Autodesk Inventor part; units mm, degrees
ref_plane "YZ Plane" through (0, 0, 0) normal (1, 0, 0) x (0, 1, 0)
ref_plane "XZ Plane" through (0, 0, 0) normal (0, 1, 0) x (-1, 0, 0)
ref_plane "XY Plane" through (0, 0, 0) normal (0, 0, 1) x (1, 0, 0)
sketch "Sketch1" plane through (0, 0, 0) normal (0, 0, 1) x (1, 0, 0)
  circle A0 centre (-3.6979, 7.9302) radius 2.5 construction
  circle A1 centre (3.6979, -7.9302) radius 2.5 construction
  line L0 (-8.2294, 5.8171) -> (-0.8336, -10.0433) construction
  arc A2 (-0.8336, -10.0433) -> (8.2294, -5.8171) centre (3.6979, -7.9302) ccw construction
  line L1 (8.2294, -5.8171) -> (0.8336, 10.0433) construction
  arc A3 (0.8336, 10.0433) -> (-8.2294, 5.8171) centre (-3.6979, 7.9302) ccw construction
  circle A4 centre (78.5293, 90.1574) radius 2.5 construction
  circle A5 centre (94.3897, 82.7616) radius 2.5 construction
  line L2 (76.4162, 85.6259) -> (92.2766, 78.2301) construction
  arc A6 (92.2766, 78.2301) -> (96.5028, 87.2931) centre (94.3897, 82.7616) ccw construction
  line L3 (96.5028, 87.2931) -> (80.6424, 94.689) construction
  arc A7 (80.6424, 94.689) -> (76.4162, 85.6259) centre (78.5293, 90.1574) ccw construction
  circle A8 centre (-75.543, 162.0025) radius 75 construction
  line L4 (112.457, 50.5739) -> (112.457, -27.9975) construction
  line L5 (107.457, -32.9975) -> (39.927, -32.9975) construction
  line L6 (-75.543, 162.0025) -> (58.8073, 27.6522) construction
  line L7 (54.2111, 23.056) -> (63.4035, 32.2484)
  line L8 (70.4745, 32.2484) -> (91.6877, 11.0352)
  line L9 (54.2111, 15.985) -> (75.4243, -5.2282)
  line L10 (75.4243, -12.2993) -> (70.027, -17.6966)
  line L11 (98.7588, 11.0352) -> (104.1561, 16.4325)
  line L12 (-0.8336, -10.0433) -> (-8.2294, 5.8171)
  line L13 (80.6424, 94.689) -> (96.5028, 87.2931)
  arc A9 (-5.811, 12.4617) -> (73.9978, 92.2705) centre (-75.543, 162.0025) ccw
  line L14 (-3.6979, 7.9302) -> (3.6979, -7.9302) construction
  line L15 (78.5293, 90.1574) -> (94.3897, 82.7616) construction
  line L16 (65.9977, -19.1366) -> (3.2042, -12.9058)
  line L17 (105.5961, 20.4618) -> (99.3653, 83.2553)
  arc A10 (75.4243, -12.2993) -> (75.4243, -5.2282) centre (71.8887, -8.7638) ccw
  arc A11 (54.2111, 23.056) -> (54.2111, 15.985) centre (57.7466, 19.5205) ccw
  arc A12 (70.4745, 32.2484) -> (63.4035, 32.2484) centre (66.939, 28.7129) ccw
  arc A13 (91.6877, 11.0352) -> (98.7588, 11.0352) centre (95.2233, 14.5708) ccw
  arc A14 (104.1561, 16.4325) -> (105.5961, 20.4618) centre (100.6206, 19.9681) ccw
  arc A15 (99.3653, 83.2553) -> (96.5028, 87.2931) centre (94.3897, 82.7616) ccw
  arc A16 (80.6424, 94.689) -> (73.9978, 92.2705) centre (78.5293, 90.1574) ccw
  arc A17 (-5.811, 12.4617) -> (-8.2294, 5.8171) centre (-3.6979, 7.9302) ccw
  arc A18 (-0.8336, -10.0433) -> (3.2042, -12.9058) centre (3.6979, -7.9302) ccw
  arc A19 (65.9977, -19.1366) -> (70.027, -17.6966) centre (66.4914, -14.1611) ccw
  point P0 (0, 0)
  point P1 (79.4008, -9.1758)
  point P2 (50.6755, 19.5205)
  point P3 (66.939, 35.784)
  point P4 (95.2233, 7.4997)
  point P5 (78.9598, -8.7638)
  point P6 (68.3532, -19.3704)
  point P7 (105.8299, 18.1063)
  point P8 (0.37, -12.6245)
  point P9 (76.0422, 96.8341)
  point P10 (99.084, 86.0895)
  point P11 (-10.3746, 10.4173)
  point P12 (-4.5315, -2.1131)
  point P13 (88.5726, 90.991)
  dimension "d56" = 190
  dimension "d64" = 23
  dimension "d65" = 40
  dimension "d67" = 165
  dimension "d68" = 15
  dimension "d69" = 15
  dimension "d70" = 20
  dimension "d73" = 5
extrude "Extrusion1" add sketch "Sketch1" along normal blind 10
sketch "Sketch2" plane through (0, 0, 10) normal (0, 0, 1) x (1, 0, 0)
  circle A0 centre (3.6979, -7.9302) radius 2.067
  circle A1 centre (-3.6979, 7.9302) radius 2.067
  circle A2 centre (94.3897, 82.7616) radius 2.067
  circle A3 centre (78.5293, 90.1574) radius 2.067
  point P0 (0, 0)
hole "Hole1" at (78.5293, 90.1574, 10) at (94.3897, 82.7616, 10) at (-3.6979, 7.9302, 10) at (3.6979, -7.9302, 10) direction (0, 0, -1) diameter 5 end through all
sketch "Sketch4" plane through (0, 0, 10) normal (0, 0, 1) x (1, 0, 0)
  circle A0 centre (-3.6979, 7.9302) radius 2.5
  circle A1 centre (78.5293, 90.1574) radius 2.5
  circle A2 centre (94.3897, 82.7616) radius 2.5
  circle A3 centre (3.6979, -7.9302) radius 2.5
  line L0 (-75.543, 162.0025) -> (25.98, 17.0126) construction
  line L1 (-75.543, 162.0025) -> (-3.6979, 7.9302) construction
  line L2 (78.5293, 90.1574) -> (-75.543, 162.0025) construction
  line L3 (-75.543, 162.0025) -> (69.4469, 60.4795) construction
  circle A4 centre (-75.543, 162.0025) radius 75
  point P0 (0, 0)
  dimension "d27" = 10
  dimension "d28" = 10
  dimension "d71" = 177
  dimension "d72" = 177
hole "Hole2" at (25.98, 17.0126, 10) at (69.4469, 60.4795, 10) direction (0, 0, -1) diameter 10 end through all
sketch "Sketch6" plane through (0, 0, 10) normal (0, 0, 1) x (1, 0, 0)
  line L0 (25.98, 17.0126) -> (10.8257, 6.4014) construction
  line L1 (25.98, 17.0126) -> (41.1343, 27.6238) construction
  line L2 (25.98, 17.0126) -> (19.0971, 26.8424) construction
  line L3 (69.4469, 60.4795) -> (58.8357, 45.3252) construction
  line L4 (69.4469, 60.4795) -> (80.0581, 75.6338) construction
  line L5 (69.4469, 60.4795) -> (59.6171, 67.3624) construction
  arc A0 (-5.811, 12.4617) -> (73.9978, 92.2705) centre (-75.543, 162.0025) ccw
  circle A1 centre (69.4469, 60.4795) radius 5
  circle A2 centre (25.98, 17.0126) radius 5
  point P0 (0, 0)
  point P1 (76.0422, 96.8341)
  point P2 (-10.3746, 10.4173)
  dimension "d29" = 18.5
  dimension "d30" = 18.5
  dimension "d38" = 18.5
  dimension "d39" = 18.5
hole "Hole3" at (10.8257, 6.4014, 10) at (41.1343, 27.6238, 10) at (58.8357, 45.3252, 10) at (80.0581, 75.6338, 10) direction (0, 0, -1) diameter 4.134 end through all
sketch "Sketch7" plane through (0, 0, 10) normal (0, 0, 1) x (1, 0, 0)
  arc A0 (50.3958, 16.2647) -> (52.016, 14.6445) centre (51.5594, 15.8082) ccw
  arc A1 (56.0526, 10.6079) -> (57.6728, 8.9877) centre (57.2163, 10.1513) ccw
  arc A2 (61.7095, 4.951) -> (63.3297, 3.3308) centre (62.8731, 4.4945) ccw
  arc A3 (67.3663, -0.7058) -> (68.9865, -2.326) centre (68.53, -1.1624) ccw
  arc A4 (71.815, 34.4435) -> (70.1948, 36.0637) centre (70.6513, 34.9001) ccw
  arc A5 (77.4718, 28.7867) -> (75.8516, 30.4069) centre (76.3082, 29.2432) ccw
  arc A6 (83.1287, 23.1298) -> (81.5085, 24.75) centre (81.965, 23.5864) ccw
  arc A7 (88.7855, 17.473) -> (87.1653, 19.0932) centre (87.6219, 17.9295) ccw
  arc A8 (63.5065, 35.8869) -> (61.8863, 34.2668) centre (63.0499, 34.7233) ccw
  arc A9 (52.1927, 24.5732) -> (50.5726, 22.953) centre (51.7362, 23.4096) ccw
  point P0 (0, 0)
hole "Hole4" at (51.7362, 23.4096, 10) at (63.0499, 34.7233, 10) at (51.5594, 15.8082, 10) at (57.2163, 10.1513, 10) at (62.8731, 4.4945, 10) at (70.6513, 34.9001, 10) at (76.3082, 29.2432, 10) at (81.965, 23.5864, 10) at (68.53, -1.1624, 10) at (87.6219, 17.9295, 10) direction (0, 0, -1) diameter 2.5 end through all
properties part number "motorplate"
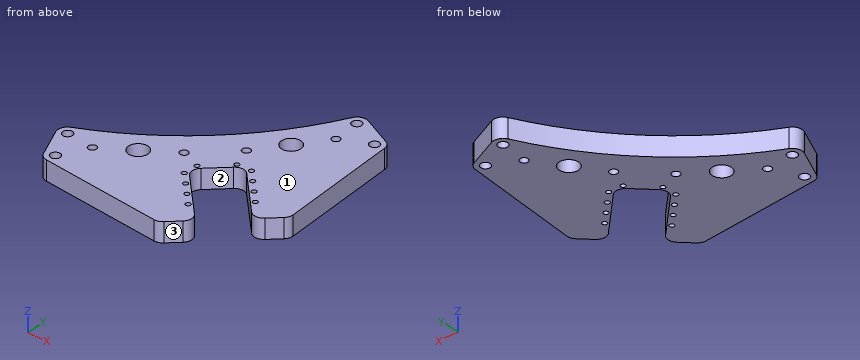
Here's how the part is built. I have some questions about the finished solid (model axes, mm). Face numbers are marked on the shaded views. Give positions to 0.01 mm unless a question says otherwise; leave off trailing zeros. Order: outer loops, then holes, each group sorted by start corner. A loop starts at its lowest first (then second) coordinate and runs counter-clockwise, first axis right, second up. Notation, with made-up numbers: (4, 4) -> (30, 4) arc R31 ccw to (30, 40) -> close; hole circle Ø5 at (36.25, -19.75). An arc over 180 degrees is marked (long way). One line per item, written item: value. Start each with the question number.
1. Imagine slicing it at B-B, the plane x = 23. List the corners of the cut face in (y, z) for me, plus the area to 3 significant figures.
2. We'd pull the mould along X, two halves only. Please class the marked faces 1, 2 and 3: released by +X, released by -X, zero draft, split by the parting line, or undercut.
3. Imagine slicing it at A-A, the plane y = 61. List the corners of the cut face in (x, z) for me.
4. Imagine slicing it at C-C, the plane z = 3.5. Count the separate pieces of the cut face and the enclosed holes in it, plus the area to 3 significant figures.
5. Will these pins go through, and if not, where does the flat tip stop? pin 1 Ø1 at (x, z) = (15, 2) entering from +Y; pin 2 Ø5.5 at (x, y) = (41.13, 27.62) entering from +Z; pin 3 Ø6 at (y, z) = (-6.5, 7.5) entering from +X; pin 4 Ø6 at (x, z) = (31.5, 8) entering from -Y.
6. I need wall thicknesses on probe 1 along Y at (x, z) = (80, 1.25); probe 2 along Y at (x, z) = (74.5, 5); probe 3 along X at (y, z) = (10, 6). Which ranges of each line are inside material? Lowest first, please. Write a range as from..to.
Values follow:
1. outline: (-14.87, 0) -> (13, 0) -> (13, 10) -> (-14.87, 10) -> close; (21.03, 0) -> (29.66, 0) -> (29.66, 10) -> (21.03, 10) -> close
1. area: 365 mm2
2. face 1: zero draft
2. face 2: undercut
2. face 3: released by +X
3. outline: (54.93, 0) -> (64.47, 0) -> (64.47, 10) -> (54.93, 10) -> close; (74.42, 0) -> (101.57, 0) -> (101.57, 10) -> (74.42, 10) -> close
4. separate pieces: 1
4. enclosed holes: 20
4. area: 5,980 mm2
5. pin 1: stops at y = 24.39
5. pin 2: stops at z = 10
5. pin 3: stops at x = 76.89
5. pin 4: stops at y = -16.01
6. probe 1: y = 22.72..73.57, 77.7..88.14, 92.18..94.94
6. probe 2: y = -13.22..-4.3, 28.22..93.12
6. probe 3: x = -8.25..-5.1, -2.3..55.98, 58.46..60.2, 93.2..97.25
